Source: CAD feature listing. Evaluate the final solid. Frame: model axes, mm. A direction names the side the tool comes from. Round coordinates to 2 decimals unless told otherwise and drop trailing zeros. Order: outer loops, then holes, each group sorted by start corner. A loop starts at its lowest first (then second) coordinate and runs counter-clockwise, first axis right, second up. Notation, with made-up numbers: (5, 15) - (41, 15) arc R22 cw to (41, 52) - close; hole circle Ø11 at (20, 68.25). An arc over 180 degrees is marked (long way). Use one line per item in the form item = value. Start each with the question number.
Q1. Cut plane A-A, the plane z = 19.75. Return the cut outline in (x, y), and give its area (3 significant figures).
Q2. Cut plane C-C, the plane x = 9. Return the cut outline in (y, z).
Q3. Cut plane B-B, the plane y = 23.5. Return the cut outline in (x, z), and give its area (3 significant figures).
Q4. Pin query (flat end, axial travel): pin 1 Ø9.5 at (x, y) = (9.5, 22.5) entering from +Z. Return the tip coordinate at first contact, or that it passes through.
Q5. Draft query along X for faces 1 (the flat face through (22, 15, 18)), 2 (the flat face through (12, 16, 0)), 3 (the flat face through (3, 15, 18)), 4 (the flat face through (25, 15, 14)). Return one class per face: released by +X, released by -X, zero draft, split by the parting line, or undercut.
Q6. Ray query, line 1 (X direction, y = 19.5, z = 12); line 2 (Z direction, x = 15, y = 22.5). Return the intervals inside material, ascending. Write a range as [from, to].
Q7. Set-up query: faces 5 (the flat face through (12, 15, 9)), 6 (the flat face through (12, 0, 8)). Return all of +Z, -Z, +X, -X, +Y, -Y with unobstructed straight access to the full face (end or side cutting, diameter ignored); none if empty.
from build123d import *

# Parameters (mm, degrees)
F0_W     = 25
F0_H     = 31
F1_DEPTH = 28
F3_W     = 19
F3_H     = 19
F4_DEPTH = 31.001


with BuildPart() as f1:
    # F0 (on Top) → F1 (new body)
    with BuildSketch(Plane.XY):
        with Locations((12.5, 15.5)):
            Rectangle(F0_W, F0_H)
    extrude(amount=F1_DEPTH)

    # F3 (on face) → F4 (cut, through all)
    with BuildSketch(Plane.XZ):
        with Locations((12.500027, 18.500176)):
            Rectangle(F3_W, F3_H)
    extrude(amount=-F4_DEPTH, mode=Mode.SUBTRACT)


solid = f1.part
Completed:
q1.outline = (0, 0) - (3, 0) - (3, 31) - (0, 31) - close; (22, 0) - (25, 0) - (25, 31) - (22, 31) - close
q1.area = 186 mm2
q2.outline = (0, 0) - (31, 0) - (31, 9) - (0, 9) - close
q3.outline = (0, 0) - (25, 0) - (25, 28) - (22, 28) - (22, 9) - (3, 9) - (3, 28) - (0, 28) - close
q3.area = 339 mm2
q4.pin_1 = 9
q5.face_1 = undercut
q5.face_2 = zero draft
q5.face_3 = undercut
q5.face_4 = released by +X
q6.line_1 = [0, 3], [22, 25]
q6.line_2 = [0, 9]
q7.face_5 = +Z, +Y, -Y
q7.face_6 = +Z, -Z, +X, -X, -Y
